The listing builds one solid part. Answer for the finished solid, in the listing's coordinates (mm). A direction names the side the tool comes from. Coordinates: 2 decimals unless noted, no trailing zeros. Order: outer loops, then holes, each group sorted by start corner. A loop starts at its lowest first (then second) coordinate and runs counter-clockwise, first axis right, second up. Notation, with made-up numbers: (-15.5, 31) -> (-4.5, 31) arc R24 cw to (-4.5, 70) -> close; hole circle Ø6 at (9, -24.75). An arc over 180 degrees is marked (long way). Write item = value, one per line.
from build123d import *

# Parameters (mm, degrees)
SKETCH001_R                          = 4
SKETCH001_R_2                        = 1.4
SKETCH001_R_3                        = 2.75
EXTRUDE001_DEPTH                     = 25
SKETCH002_AS_DRAWN_W                 = 15
SKETCH002_AS_DRAWN_H                 = 13
SKETCH002_AS_DRAWN_R                 = 3.35
EXTRUDE002_DEPTH                     = 3
EXTRUDE002_ONTO_SKETCH002_ROLL_ANGLE = 90
SKETCH_R                             = 1.9
SKETCH_R_2                           = 23
SKETCH_R_3                           = 1.85
EXTRUDE_DEPTH                        = 3
CHAMFER_SIZE                         = 0.6


with BuildPart() as extrude001:
    # Sketch001 → Extrude001 (new body)
    with BuildSketch(Plane.XY):
        with Locations((-50.25, -47.25)):
            Circle(SKETCH001_R)
        with Locations((-50.25, -47.25)):
            Circle(SKETCH001_R_2, mode=Mode.SUBTRACT)
        with Locations((50.25, 47.25)):
            Circle(SKETCH001_R)
        with Locations((50.25, 47.25)):
            Circle(SKETCH001_R_2, mode=Mode.SUBTRACT)
        with Locations((-50.25, 47.25)):
            Circle(SKETCH001_R)
        with Locations((-50.25, 47.25)):
            Circle(SKETCH001_R_2, mode=Mode.SUBTRACT)
        with Locations((25.25, -42.25)):
            Circle(SKETCH001_R)
        with Locations((25.25, -42.25)):
            Circle(SKETCH001_R_2, mode=Mode.SUBTRACT)
        with Locations((51.25, -51.75)):
            Circle(SKETCH001_R_3)
        with Locations((-14.75, -39.25)):
            Circle(SKETCH001_R)
        with Locations((-14.75, -39.25)):
            Circle(SKETCH001_R_2, mode=Mode.SUBTRACT)
    extrude(amount=EXTRUDE001_DEPTH)


with BuildPart() as extrude002:
    # Sketch002 as drawn → Extrude002 (new)
    with BuildSketch(Plane.XY):
        with Locations((0, 6.5)):
            Rectangle(SKETCH002_AS_DRAWN_W, SKETCH002_AS_DRAWN_H)
        with Locations((0, 7)):
            Circle(SKETCH002_AS_DRAWN_R, mode=Mode.SUBTRACT)
    extrude(amount=-EXTRUDE002_DEPTH)


with BuildPart() as extrude002_1:
    # Extrude002 onto Sketch002 roll: moved
    add(extrude002.part.rotate(Axis((0, 0, 0), (1, 0, 0)), EXTRUDE002_ONTO_SKETCH002_ROLL_ANGLE))


with BuildPart() as extrude002_2:
    # Extrude002 onto Sketch002 placement: moved
    add(extrude002_1.part)


with BuildPart() as extrude002_3:
    # Extrude002 placement: moved
    add(extrude002_2.part.moved(Location((32, 61, 2))))


with BuildPart() as chamfer_body:
    # Sketch → Extrude (new body)
    with BuildSketch(Plane.XY):
        Polygon((55.5, 55), (55.5, -55), (-55.5, -55), (-55.5, 55), (24.5, 55), (24.5, 65), (39.5, 65), (39.5, 55), align=None)
        with Locations((-50.25, -47.25)):
            Circle(SKETCH_R, mode=Mode.SUBTRACT)
        Circle(SKETCH_R_2, mode=Mode.SUBTRACT)
        with Locations((-39.25, 47.25)):
            Circle(SKETCH_R_3, mode=Mode.SUBTRACT)
        with Locations((0.75, 47.25)):
            Circle(SKETCH_R_3, mode=Mode.SUBTRACT)
        with Locations((-39.25, 32.25)):
            Circle(SKETCH_R_3, mode=Mode.SUBTRACT)
        with Locations((0.75, 32.25)):
            Circle(SKETCH_R_3, mode=Mode.SUBTRACT)
        with Locations((10.75, 44.25)):
            Circle(SKETCH_R_3, mode=Mode.SUBTRACT)
        with Locations((40.75, 44.25)):
            Circle(SKETCH_R_3, mode=Mode.SUBTRACT)
        with Locations((10.75, 32.25)):
            Circle(SKETCH_R_3, mode=Mode.SUBTRACT)
        with Locations((40.75, 32.25)):
            Circle(SKETCH_R_3, mode=Mode.SUBTRACT)
        with Locations((50.25, 47.25)):
            Circle(SKETCH_R, mode=Mode.SUBTRACT)
        with Locations((-50.25, 47.25)):
            Circle(SKETCH_R, mode=Mode.SUBTRACT)
        with Locations((25.25, -42.25)):
            Circle(SKETCH_R, mode=Mode.SUBTRACT)
        with Locations((-14.75, -39.25)):
            Circle(SKETCH_R, mode=Mode.SUBTRACT)
        with Locations((-37.25, -7.25)):
            Circle(SKETCH_R_3, mode=Mode.SUBTRACT)
        with Locations((-37.25, -47.25)):
            Circle(SKETCH_R_3, mode=Mode.SUBTRACT)
    extrude(amount=EXTRUDE_DEPTH)

    # Fusion: union Extrude001, Extrude002
    add(extrude001.part)
    add(extrude002_3.part)

    # Chamfer
    chamfer_edges = [chamfer_body.edges().sort_by_distance(p)[0] for p in [
        (32, 61, 3),
        (32, 64, 3),
        (-54.25, -47.25, 3),
        (-18.75, -39.25, 3),
        (21.25, -42.25, 3),
        (-54.25, 47.25, 3),
        (46.25, 47.25, 3),
    ]]
    chamfer(chamfer_edges, length=CHAMFER_SIZE)


solid = chamfer_body.part
Q1. A tool of negligible diameter and unlimited length cuts with its end or side. For faces 4 (the face through (-50, -49, 25)), 5 (the face through (24.729, -38.284, 14.15)), 6 (the face through (30, 61, 12)), 7 (the face through (32, 62, 15)), 8 (the face through (39.3, 43.1, 1.5)), from which of +Z, -Z, +X, -X, +Y, -Y can it reach the whole face along a straight path? Write none if from no direction.
The answers:
face_4 = +Z, +X, -X, +Y, -Y
face_5 = +Z
face_6 = +Z, +X, -X
face_7 = +Z, +X, -X, +Y
face_8 = +Z, -Z
Q2. Section C-C, the plane x = 10.75 is taken. Give the vertices of the cut face in (y, z), plus the area to 3 significant figures.
The answers:
outline = (-55, 0) -> (-20.33, 0) -> (-20.33, 3) -> (-55, 3) -> close; (20.33, 0) -> (30.4, 0) -> (30.4, 3) -> (20.33, 3) -> close; (34.1, 0) -> (42.4, 0) -> (42.4, 3) -> (34.1, 3) -> close; (46.1, 0) -> (55, 0) -> (55, 3) -> (46.1, 3) -> close
area = 186 mm2
Q3. Section D-D, the plane y = -12.5 is taken. Give the vertices of the cut face in (x, z), plus the area to 3 significant figures.
The answers:
outline = (-55.5, 0) -> (-19.31, 0) -> (-19.31, 3) -> (-55.5, 3) -> close; (19.31, 0) -> (55.5, 0) -> (55.5, 3) -> (19.31, 3) -> close
area = 217 mm2
Q4. Section A-A, the plane z = 17 is taken. Give the number of separate pieces and of enclosed holes in the cut face, plus the area to 3 significant figures.
The answers:
separate_pieces = 6
enclosed_holes = 5
area = 244 mm2
Q5. The mould has two halves that part along Y. Classify faces 1 (the face through (11.604, 42.609, 1.479)), 2 (the face through (1, -55, 1)), 3 (the face through (24.5, 62, 6)): released by +Y, released by -Y, zero draft, split by the parting line, or undercut.
The answers:
face_1 = undercut
face_2 = released by -Y
face_3 = zero draft
Q6. Each of these flat-tipped pins is pushed along its axis until it touches: pin 1 Ø3 at (x, z) = (-17.5, 6) entering from -Y; pin 2 Ø1.5 at (x, y) = (34, 62) entering from +Z; pin 3 Ø10.5 at (x, z) = (32, 9) entering from -Y. Where does it stop, or does it pass through?
The answers:
pin_1 = -43.05
pin_2 = 15
pin_3 = -45.96
Q7. Find the intervals of material crossed by line 1 along Y through (x, z) = (-39.25, 2.2); line 2 along Y through (x, z) = (0.75, 1.3); line 3 along Y through (x, z) = (40.75, 1.25), in increasing order.
The answers:
line_1 = -55 to 30.4, 34.1 to 45.4, 49.1 to 55
line_2 = -55 to -22.99, 22.99 to 30.4, 34.1 to 45.4, 49.1 to 55
line_3 = -55 to 30.4, 34.1 to 42.4, 46.1 to 55
